```python
from build123d import *

# Parameters (mm, degrees)
SKETCH2_W           = 15.5
SKETCH2_H           = 2
SKETCH3_W           = 91
SKETCH3_H           = 79
BOSS_EXTRUDE1_DEPTH = 66.8


with BuildPart() as part:
    # Sketch1 → Revolve1 (revolve)
    with BuildSketch(Plane.XY):
        with BuildLine():
            Line((0, 0), (-7, 0))
            Line((-7, 0), (-7, 41))
            Line((-7, 41), (-13.369653316, 41))
            Line((-13.369653316, 41), (-15.5, 71.401844965))
            Line((-15.5, 71.401844965), (-15.5, 77))
            ThreePointArc((-15.5, 77), (-14.328427125, 79.828427125), (-11.5, 81))
            Line((-11.5, 81), (0, 81))
            Line((0, 81), (0, 0))
        make_face()
    revolve(axis=Axis((0, 0, 0), (0, -1, 0)))

    # Sketch2 → Revolve2 (revolve)
    with BuildSketch(Plane.XY):
        with Locations((-14.75, 20.05)):
            Rectangle(SKETCH2_W, SKETCH2_H)
    revolve(axis=Axis((0, 0, 0), (0, 1, 0)))

    # Sketch3 → Boss-Extrude1 (add)
    with BuildSketch(Plane.XZ):
        Rectangle(SKETCH3_W, SKETCH3_H)
    extrude(amount=BOSS_EXTRUDE1_DEPTH)


solid = part.part
```
The model under review builds one solid part; all positions refer to its coordinate system, in mm. A direction names the side the tool comes from. Coordinates: 2 decimals unless noted, no trailing zeros. Write each loop counter-clockwise with the first axis right and the second up, starting at its lowest first coordinate (ties: lowest second). Pieces come first, ordered by that corner, then holes. Notation, with made-up numbers: (57, 9.25) -> (95, 9.25) arc R12 ccw to (95, 20.25) -> close; hole circle Ø4 at (51.5, 1.5). An arc over 180 degrees is marked (long way). One line per item, written item: value. Start each with the question number.
Q1. Add section C-C, the plane x = 17.5. Give the boundary of the cut face in (y, z), then the cut area to 3 significant figures.
Q2. For faces 1 (the face through (2.018, 74.24, -15.368)), 2 (the face through (5.3, 19.05, 5.3)), 3 (the face through (-1, -66.8, 1)), list the 3-axis set-ups (+Z, -Z, +X, -X, +Y, -Y) from which the entire face can be reached by the end or side of a thin tool; tool diameter is ignored.
Q3. The part is to be moulded in two halves that separate along Y. For faces 4 (the face through (0, 81, 0)), 5 (the face through (-6.466, 31.165, 2.681)), 6 (the face through (-10.382, 20.064, -19.961)), say which applies: +Y half, -Y half, draft (parallel to the pull), parting line (faces both ways), or undercut.
Q4. To check wall thickness, follow probe 1 along Y at (x, z) = (-2.5, -7); probe 2 along Y at (x, z) = (-11.5, 12); probe 3 along Y at (x, z) = (39.5, 31). State the ranges of each line that lie inside material, in increasing order.
Q5. Add section B-B, the plane z = 0. Give the boundary of the cut face in (x, y), then the cut area to 3 significant figures.
Q6. Add section D-D, the plane y = 68.5. Give the boundary of the cut face in (x, z).
Q7. Add section A-A, the plane x = 0. Give the boundary of the cut face in (y, z).
Q8. Clearance check with flat-ended pins moving along their axes: P1, Ø1, axis at x = 14, z = 1, coming from the +Y side; P2, Ø4, axis at x = 14.5, z = -14, coming from the +Y side; P3, Ø8, axis at x = 1, y = 41.5, coming from the +Z side. State where each tip first meets the part, or that it passes through.
Response:
1. outline: (-66.8, -39.5) -> (0, -39.5) -> (0, 39.5) -> (-66.8, 39.5) -> close; (19.05, -14.14) -> (21.05, -14.14) -> (21.05, 14.14) -> (19.05, 14.14) -> close
1. area: 5,330 mm²
2. face 1: +Y
2. face 2: none
2. face 3: +Z, -Z, +X, -X, -Y
3. face 4: +Y half
3. face 5: undercut
3. face 6: draft
4. probe 1: -66.8 to 0, 19.05 to 21.05, 41 to 81
4. probe 2: -66.8 to 0, 19.05 to 21.05
4. probe 3: -66.8 to 0
5. outline: (-45.5, -66.8) -> (45.5, -66.8) -> (45.5, 0) -> (7, 0) -> (7, 19.05) -> (22.5, 19.05) -> (22.5, 21.05) -> (7, 21.05) -> (7, 41) -> (13.37, 41) -> (15.5, 71.4) -> (15.5, 77) arc R4 ccw to (11.5, 81) -> (-11.5, 81) arc R4 ccw to (-15.5, 77) -> (-15.5, 71.4) -> (-13.37, 41) -> (-7, 41) -> (-7, 21.05) -> (-22.5, 21.05) -> (-22.5, 19.05) -> (-7, 19.05) -> (-7, 0) -> (-45.5, 0) -> close
5. area: 7,880 mm²
6. outline: circle Ø30.59 at (0, 0)
7. outline: (-66.8, -39.5) -> (0, -39.5) -> (0, -7) -> (19.05, -7) -> (19.05, -22.5) -> (21.05, -22.5) -> (21.05, -7) -> (41, -7) -> (41, -13.37) -> (71.4, -15.5) -> (77, -15.5) arc R4 ccw to (81, -11.5) -> (81, 11.5) arc R4 ccw to (77, 15.5) -> (71.4, 15.5) -> (41, 13.37) -> (41, 7) -> (21.05, 7) -> (21.05, 22.5) -> (19.05, 22.5) -> (19.05, 7) -> (0, 7) -> (0, 39.5) -> (-66.8, 39.5) -> close
8. P1: y = 80.44
8. P2: y = 21.05
8. P3: z = 13.68
